Input: part model. Units: mm. Frame: model coordinates. Face numbers are marked on the shaded views. A direction names the side the tool comes from. Give positions to 0.01 mm unless a question says otherwise; leave off trailing zeros. Loops run counter-clockwise (first coordinate to the right, second up) from the corner with the lowest first, then second, coordinate; pieces in that order, holes last.
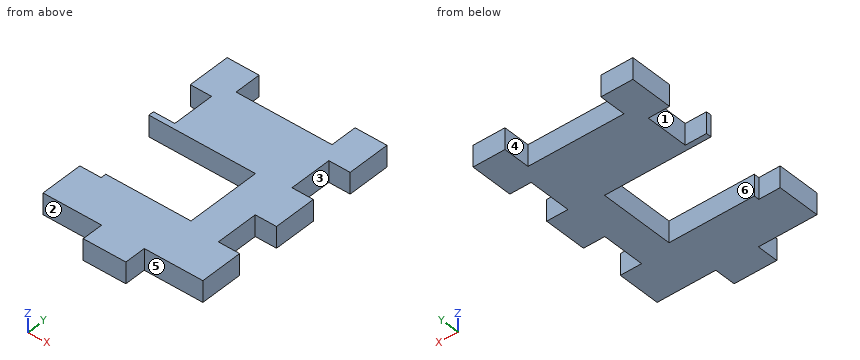
from build123d import *

# Parameters (mm, degrees)
SKETCH1_W           = 47.625
SKETCH1_H           = 63.5
BOSS_EXTRUDE1_DEPTH = 6.35
SKETCH2_W           = 12.7
SKETCH2_H           = 12.7
BOSS_EXTRUDE2_DEPTH = 6.35
SKETCH3_W           = 6.35
SKETCH3_H           = 12.7
CUT_EXTRUDE1_DEPTH  = 85.77904001
LPATTERN1_COUNT     = 2
LPATTERN1_PITCH     = 25.4
SKETCH4_W           = 50.8
SKETCH4_H           = 22.225
SERVO_CUT_DEPTH     = 85.77904001
SKETCH5_W           = 28.575
SKETCH5_H           = 15.875
CUT_EXTRUDE2_DEPTH  = 85.77904001


with BuildPart() as part:
    # Sketch1 → Boss-Extrude1 (new body)
    with BuildSketch(Plane.XY):
        with Locations((23.8125, 38.1)):
            Rectangle(SKETCH1_W, SKETCH1_H)
    extrude(amount=BOSS_EXTRUDE1_DEPTH)

    # Sketch2 → Boss-Extrude2 (add)
    with BuildSketch(Plane.XY.offset(6.35)):
        with Locations((23.8125, 6.35)):
            Rectangle(SKETCH2_W, SKETCH2_H)
    extrude(amount=-BOSS_EXTRUDE2_DEPTH)

    # Sketch3 → Cut-Extrude1 (cut, through all)
    with BuildSketch(Plane.XY.offset(6.35)):
        with Locations((3.175, 25.4)):
            Rectangle(SKETCH3_W, SKETCH3_H)
        with Locations((44.45, 25.4)):
            Rectangle(SKETCH3_W, SKETCH3_H)
    cut_extrude1 = extrude(amount=-CUT_EXTRUDE1_DEPTH, mode=Mode.SUBTRACT)

    # LPattern1: Cut-Extrude1 ×2
    with Locations(*[(0, i * LPATTERN1_PITCH, 0) for i in range(1, LPATTERN1_COUNT)]):
        add(cut_extrude1, mode=Mode.SUBTRACT)

    # Sketch4 → Servo Cut (cut, through all)
    with BuildSketch(Plane.XY.offset(6.35)):
        with Locations((6.35, 31.75)):
            Rectangle(SKETCH4_W, SKETCH4_H)
    extrude(amount=-SERVO_CUT_DEPTH, mode=Mode.SUBTRACT)

    # Sketch5 → Cut-Extrude2 (cut, through all)
    with BuildSketch(Plane.XY.offset(6.35)):
        with Locations((23.8125, 69.85)):
            Rectangle(SKETCH5_W, SKETCH5_H)
    extrude(amount=-CUT_EXTRUDE2_DEPTH, mode=Mode.SUBTRACT)


solid = part.part
(1) Ray query, probe 1 along Y at (x, z) = (42.5, 2.25); probe 2 along Y at (x, z) = (9, 1.5); probe 3 along Y at (x, z) = (26, 2). Return the intervals inside material, ascending.
Values follow:
probe 1: y = 6.35 to 19.05, 31.75 to 44.45, 57.15 to 69.85
probe 2: y = 6.35 to 20.64, 42.86 to 69.85
probe 3: y = 0 to 20.64, 42.86 to 61.91
(2) Cut plane B-B (y = 63.5). Return the cut outline in (x, z) (3 decimals), and give its area (3 significant figures).
Values follow:
outline: (0, 0) - (9.525, 0) - (9.525, 6.35) - (0, 6.35) - close; (38.1, 0) - (47.625, 0) - (47.625, 6.35) - (38.1, 6.35) - close
area: 121 mm2
(3) Reachability of the marked faces 1, 2 and 3 from +Z, -Z, +X, -X, +Y, -Y: full face, straight path, thin tool, end or side. Return the list, or none.
Values follow:
face 1: +Z, -Z, -X
face 2: +Z, -Z, -X, -Y
face 3: +Z, -Z, +X
(4) Cut plane A-A (x = 8). Return the cut outline in (y, z), and give its area (3 significant figures).
Values follow:
outline: (6.35, 0) - (20.64, 0) - (20.64, 6.35) - (6.35, 6.35) - close; (42.86, 0) - (69.85, 0) - (69.85, 6.35) - (42.86, 6.35) - close
area: 262 mm2
(5) Mould query, pull axis Y, two halves, no side actions, for the marked faces 4, 5 and 6. Classes: +Y half, -Y half, draft (parallel to the pull), parting line (faces both ways), or undercut.
Values follow:
face 4: draft
face 5: -Y half
face 6: undercut
(6) Cut plane D-D (y = 41). Return the cut outline in (x, z) (3 decimals), and give its area (3 significant figures).
Values follow:
outline: (31.75, 0) - (47.625, 0) - (47.625, 6.35) - (31.75, 6.35) - close
area: 101 mm2
(7) Pin query (flat end, axial travel): pin 1 Ø1.9 at (y, z) = (52, 4) entering from +X (3 decimals); pin 2 Ø1.5 at (x, z) = (34, 4) entering from +Y; pin 3 Ø1.9 at (x, z) = (38, 3) entering from -Y. Return the tip coordinate at first contact, or that it passes through.
Values follow:
pin 1: stops at x = 41.275
pin 2: stops at y = 61.91
pin 3: stops at y = 6.35
